```python
from build123d import *

# Parameters (mm, degrees)
F1_DEPTH = 15.875
F2_R     = 0.762
F3_R     = 1.98374
F4_R     = 3.69316
F5_W     = 6.707656
F5_H     = 2.38125
F6_DEPTH = 1.70942
F7_R     = 1.35255
F8_DEPTH = 1.70942


with BuildPart() as f1:
    # F0 (on Top) → F1 (new body)
    with BuildSketch(Plane.XY):
        Polygon((0, 0), (0, -11.952478), (1.70942, -11.952478), (1.70942, 1.70942), (-9.92124, 1.70942), (-9.92124, 0), align=None)
    extrude(amount=F1_DEPTH)

    # F2
    f2_edges = [f1.edges().sort_by_distance(p)[0] for p in [
        (-9.92124, 0.85471, 15.875),
        (-9.92124, 0.85471, 0),
        (0.85471, -11.952478, 0),
        (0.85471, -11.952478, 15.875),
    ]]
    fillet(f2_edges, radius=F2_R)

    # F3
    f3_edges = [f1.edges().sort_by_distance(p)[0] for p in [
        (0, 0, 7.9375),
    ]]
    fillet(f3_edges, radius=F3_R)

    # F4
    f4_edges = [f1.edges().sort_by_distance(p)[0] for p in [
        (1.70942, 1.70942, 7.9375),
    ]]
    fillet(f4_edges, radius=F4_R)

    # F5 (on face) → F6 (cut, through all)
    with BuildSketch(Plane(origin=(0, 0, 0), x_dir=(0, -1, 0), z_dir=(-1, 0, 0))):
        with Locations((6.925068, 12.303125)):
            Rectangle(F5_W, F5_H)
        with Locations((6.925068, 3.571875)):
            Rectangle(F5_W, F5_H)
    extrude(amount=-F6_DEPTH, mode=Mode.SUBTRACT)

    # F7 (on face) → F8 (cut, through all)
    with BuildSketch(Plane.XZ):
        with Locations((-5.95249, 11.90625)):
            Circle(F7_R)
        with Locations((-5.95249, 3.96875)):
            Circle(F7_R)
    extrude(amount=-F8_DEPTH, mode=Mode.SUBTRACT)


solid = f1.part
```
The model under review builds one solid part; all positions refer to its coordinate system, in mm. A direction names the side the tool comes from. Give positions to 0.01 mm unless a question says otherwise; leave off trailing zeros. Write each loop counter-clockwise with the first axis right and the second up, starting at its lowest first coordinate (ties: lowest second). Pieces come first, ordered by that corner, then holes. Notation, with made-up numbers: (58.25, 0) -> (114.25, 0) arc R8 cw to (114.25, 10) -> close; hole circle Ø5 at (-6.75, 42.5). An arc over 180 degrees is marked (long way). Put each result on its own line as item: value.
(1) We need section D-D, the plane y = 0.75. Give the boundary of the cut face in (x, z) (3 decimals), and give its area (3 significant figures).
Results are:
outline: (-9.921, 0.762) arc R0.762 ccw to (-9.159, 0) -> (0.499, 0) -> (0.499, 15.875) -> (-9.159, 15.875) arc R0.762 ccw to (-9.921, 15.113) -> close; hole circle Ø2.705 at (-5.952, 3.969); hole circle Ø2.705 at (-5.952, 11.906)
area: 154 mm²
(2) For pin 1 Ø5 at (y, z) = (-8.5, 8.5) entering from -X; pin 2 Ø4 at (x, z) = (-4.5, 8) entering from -Y; pin 3 Ø1.4 at (x, z) = (1, 12) entering from +Y; pin 4 Ø1 at (x, y) = (-4, -2) entering from +Z, all flat-tipped, find the tip position at first contact; note any pin that passes through.
Results are:
pin 1: x = 0
pin 2: y = 0
pin 3: y = 0.92
pin 4: through
(3) To check wall thickness, follow probe 1 along X at (y, z) = (-4.75, 6.25); probe 2 along Y at (x, z) = (1, 2.5). State the ranges of each line that lie inside material, in increasing order. Write a range as from..to.
Results are:
probe 1: 0..1.71
probe 2: -11.95..-10.28, -3.57..0.19
(4) We need section C-C, the plane z = 1.75. Give the boundary of the cut face in (x, y), and give its area (3 significant figures).
Results are:
outline: (-9.92, 0) -> (-1.98, 0) arc R1.98 cw to (0, -1.98) -> (0, -11.95) -> (1.71, -11.95) -> (1.71, -1.98) arc R3.69 ccw to (-1.98, 1.71) -> (-9.92, 1.71) -> close
area: 38.2 mm²
(5) We need section A-A, the plane z = 12.75. Give the boundary of the cut face in (x, y).
Results are:
outline: (-9.92, 0) -> (-7.01, 0) -> (-7.01, 1.71) -> (-9.92, 1.71) -> close; (-4.9, 0) -> (-1.98, 0) arc R1.98 cw to (0, -1.98) -> (0, -3.57) -> (1.71, -3.57) -> (1.71, -1.98) arc R3.69 ccw to (-1.98, 1.71) -> (-4.9, 1.71) -> close; (0, -11.95) -> (1.71, -11.95) -> (1.71, -10.28) -> (0, -10.28) -> close
(6) Tool access review of faces 5 (the cylindrical face through (0.656, 0.599, 8.049)), 6 (the flat face through (0, -7, 8)), 7 (the flat face through (1, -7, 13.494)): name each direction out of +Z, -Z, +X, -X, +Y, -Y from which nothing blocks a thin tool from reaching the whole face with its end or side.
Results are:
face 5: +Z, -Z, +X, +Y
face 6: +Z, -Z, -X, -Y
face 7: +X, -X
(7) We need section B-B, the plane y = -9.75. Give the boundary of the cut face in (x, z) (1 decimal), and give its area (3 significant figures).
Results are:
outline: (0, 0) -> (1.7, 0) -> (1.7, 2.4) -> (0, 2.4) -> close; (0, 4.8) -> (1.7, 4.8) -> (1.7, 11.1) -> (0, 11.1) -> close; (0, 13.5) -> (1.7, 13.5) -> (1.7, 15.9) -> (0, 15.9) -> close
area: 19.0 mm²
(8) The part is to be moulded in two halves that separate along Z. For faces 1 (the flat face through (-9.921, 1, 8)), 2 (the flat face through (0.3, -2.3, 0)), 3 (the flat face through (0.3, -2.3, 15.875)), 4 (the flat face through (1, -10.279, 12)), say which applies: pulls with the +Z half, pulls with the -Z half, needs draft (parallel to the pull), parting line crosses it, or undercut.
Results are:
face 1: needs draft
face 2: pulls with the -Z half
face 3: pulls with the +Z half
face 4: undercut
